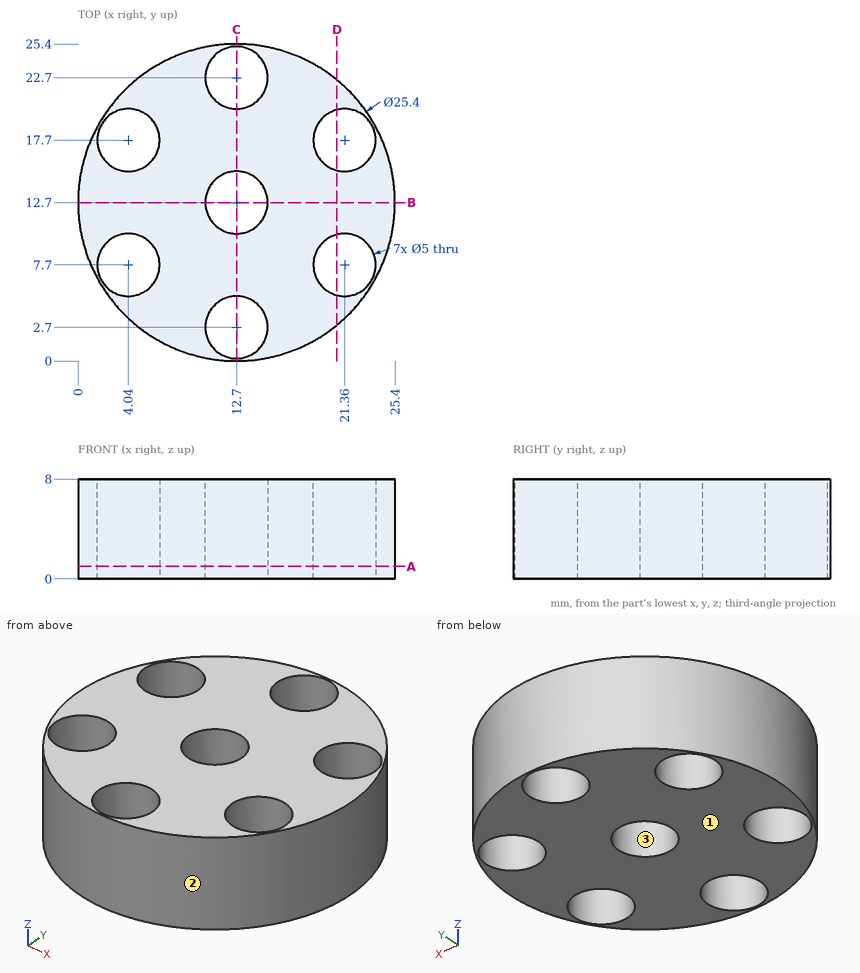
Geometry: see drawing. Coordinates: mm, zero at the bounding-box minimum. Coordinates: 2 decimals unless noted, no trailing zeros. Order: outer loops, then holes, each group sorted by start corner. A loop starts at its lowest first (then second) coordinate and runs counter-clockwise, first axis right, second up. Notation, with made-up numbers: M -35.75,60 L -7.75,60 A21 cw -7.75,73 Z; hole C -27,-33 d2. An arc over 180 degrees is marked long. Write item = value, one per line. Start each with the question number.
(1) Section C-C on x = 12.7. Output: boundary loops of the cut face in (y, z).
(2) Section D-D on x = 20.75. Output: boundary loops of the cut face in (y, z), and give its area (3 significant figures).
(3) Line query: line 1 along Y through (x, z) = (12.7, 4); line 2 along X through (y, z) = (16, 4.75) (1 decimal); line 3 along Y through (x, z) = (14.5, 0.75) (1 decimal). Output: solid intervals per line, ascending. Write a range as [from, to].
(4) Pull-direction query (X, two-part tool) for the marked faces 1, 2 and 3; classes: released by +X, released by -X, zero draft, split by the parting line, or undercut.
(5) First-contact query: P1, Ø2, axis at x = 9, z = 7, coming from the -Y side; P2, Ø2, axis at x = 9.5, z = 3.5, coming from the -Y side; P3, Ø1, axis at y = 11, z = 7, coming from the +X side. Flat tips, straight axial feed; report the tip coordinate or a pass-through.
(6) Section A-A on z = 1. Output: boundary loops of the cut face in (x, y), and give its area (3 significant figures).
(7) Section B-B on y = 12.7. Output: boundary loops of the cut face in (x, z), and give its area (3 significant figures).
Result set:
q1.outline = M 0,0 L 0.2,0 L 0.2,8 L 0,8 Z; M 5.2,0 L 10.2,0 L 10.2,8 L 5.2,8 Z; M 15.2,0 L 20.2,0 L 20.2,8 L 15.2,8 Z; M 25.2,0 L 25.4,0 L 25.4,8 L 25.2,8 Z
q2.outline = M 2.88,0 L 5.28,0 L 5.28,8 L 2.88,8 Z; M 10.12,0 L 15.28,0 L 15.28,8 L 10.12,8 Z; M 20.12,0 L 22.52,0 L 22.52,8 L 20.12,8 Z
q2.area = 79.6 mm²
q3.line_1 = [0, 0.2], [5.2, 10.2], [15.2, 20.2], [25.2, 25.4]
q3.line_2 = [0.4, 2.2], [5.9, 19.5], [23.2, 25]
q3.line_3 = [0.1, 1], [4.4, 11], [14.4, 21], [24.4, 25.3]
q4.face_1 = zero draft
q4.face_2 = split by the parting line
q4.face_3 = undercut
q5.P1 = 0.29
q5.P2 = 0.19
q5.P3 = 25.34
q6.outline = C 12.7,12.7 d25.4; hole C 4.04,7.7 d5; hole C 4.04,17.7 d5; hole C 12.7,2.7 d5; hole C 12.7,12.7 d5; hole C 12.7,22.7 d5; hole C 21.36,7.7 d5; hole C 21.36,17.7 d5
q6.area = 369 mm²
q7.outline = M 0,0 L 10.2,0 L 10.2,8 L 0,8 Z; M 15.2,0 L 25.4,0 L 25.4,8 L 15.2,8 Z
q7.area = 163 mm²
